Read the model definition and answer for the solid it produces. Units are mm, in the model's axes. A direction names the side the tool comes from. Give positions to 0.01 mm unless a question says otherwise; leave off trailing zeros. Order: outer loops, then holes, each group sorted by start corner. A loop starts at its lowest first (then second) coordinate and runs counter-clockwise, first axis right, second up. Notation, with made-up numbers: (38, 72.25) - (72, 72.25) arc R11 ccw to (72, 91.25) - close; hole circle Ø1 at (-8, 69). An arc over 180 degrees is marked (long way). Use a Markdown table: item, result. Add a question column.
1. Flat-ended cylindrical pins translate along their axes: P1, Ø3.5, axis at x = 14, y = 14, coming from the -Z side; P2, Ø1.3, axis at x = 13, y = 13.5, coming from the +Z side; P3, Ø1.9, axis at y = 5.5, z = -7, coming from the -X side. Find the tip coordinate at first contact, or state that the pin passes through.
2. Consider L1, parallel to Y at x = 14, z = -0.4; L2, parallel to Y at x = 14, z = -2.05; L3, parallel to X at y = -5, z = -2.25. Determine where each line is inside the solid, lowest interval first.
3. A cutting plane is placed at A-A on x = 14. Determine the outline of the cut face in (y, z), and give its area (3 significant figures).
4. Which of the six approach directions +Z, -Z, +X, -X, +Y, -Y give full straight-line access (tool end or side, diameter ignored) to faces 5 (the flat face through (-22.014, -7.678, -4.182)), 6 (the cylindrical face through (-11.43, 11.4, -1.97)), 7 (the cylindrical face through (24.22, 0.72, -9.29))?
5. A cutting plane is placed at B-B on y = -14. State how many separate pieces and enclosed holes the cut face has, and give its area (3 significant figures).
6. For a pull along Y with two mould halves and no side action, classify faces 1 (the cylindrical face through (18.4, 18.43, -1.97)), 2 (the flat face through (-21, 0, -12)), 3 (the cylindrical face through (14.176, -12.661, -3.586)), 4 (the flat face through (-14, 12.5, -1)) as released by +Y, released by -Y, zero draft, split by the parting line, or undercut.
7. A cutting plane is placed at C-C on x = -3.5. Determine the outline of the cut face in (y, z).
```python
from build123d import *

# Parameters (mm, degrees)
EXTRUDE_1_DEPTH           = 4
EXTRUDE_START             = -4
SKETCH_6_R                = 2.5000000000000004
SKETCH_6_R_2              = 2.4999999999999987
EXTRUDE_5_DEPTH           = 2.1
HOLE_WIZARD_1_D           = 2.7
HOLE_WIZARD_1_CBORE_D     = 4.5
HOLE_WIZARD_1_CBORE_DEPTH = 1
EXTRUDE_3_DEPTH           = 4
FILLET_1_R                = 2
CUT_EXTRUDE_1_DEPTH       = 2
SKETCH_14_R               = 3.150000000000003
CUT_EXTRUDE_4_DEPTH       = 0.8
EXTRUDE_6_DEPTH           = 3
SKETCH_11_R               = 2.399999999999999
EXTRUDE_7_DEPTH           = 5
FILLET_2_RADIUS           = 6
FILLET_2_LENGTH           = 3
FILLET_4_R                = 2
FILLET_6_R                = 0.5
CUT_EXTRUDE_2_DEPTH       = 0.4
CUT_EXTRUDE_3_DEPTH       = 0.4
CHAMFER_1_SIZE            = 2.5


with BuildPart() as part:
    # 草图1 → 凸台-拉伸1 (new body)
    with BuildSketch(Plane.XY):
        Polygon((19, -19), (11.999999999999977, -19), (11.000000000000004, -19), (11.000000000000002, -11.999999999999998), (11.999999999999977, -11.999999999999973), (11.999999999999977, 12.000000000000027), (-12.000000000000023, 12.000000000000023), (-12.000000000000023, -11.999999999999977), (-10.999999999999996, -12.000000000000002), (-10.999999999999996, -19), (-11.999999999999996, -19), (-19, -19), (-19, 19), (19, 19), align=None)
    extrude(amount=-EXTRUDE_1_DEPTH)

    # 草图6 → 凸台-拉伸5 (add)
    with BuildSketch(Plane.XY.offset(EXTRUDE_START)):
        with Locations((-14.000000000000115, 14.000000000000014)):
            Circle(SKETCH_6_R)
        with Locations((-14.000000000000112, -13.999999999999996)):
            Circle(SKETCH_6_R)
        with Locations((14.0000000000001, -13.99999999999998)):
            Circle(SKETCH_6_R_2)
        with Locations((14.000000000000096, 14.00000000000002)):
            Circle(SKETCH_6_R_2)
    extrude(amount=-EXTRUDE_5_DEPTH)

    # 孔1 (through all)
    with Locations(Plane.XY):
        with Locations((-14, 14), (14, -14), (14, 14), (-14, -14), (0, 0), (0.008296822, -0.048065229)):
            CounterBoreHole(HOLE_WIZARD_1_D / 2, HOLE_WIZARD_1_CBORE_D / 2, HOLE_WIZARD_1_CBORE_DEPTH)

    # 草图5 → 凸台-拉伸3 (add)
    with BuildSketch(Plane.ZY.offset(19)):
        Polygon((-12.000000000000004, -19.000000000000007), (-4.47e-15, -19.000000000000004), (-3.7e-16, 18.999999999999996), (-12.000000000000004, 18.999999999999993), align=None)
    extrude(amount=EXTRUDE_3_DEPTH)

    # 圆角1
    # the kernel refuses this fillet: 2 mm, written as the material it adds along each edge
    with BuildSketch(Plane(origin=(11.999999999999977, 12.000000000000027, 0), x_dir=(-1, 0, 0), z_dir=(0, 0, -1)), Plane(origin=(-12.000000000000023, 12.000000000000023, 0), x_dir=(0, -1, 0), z_dir=(0, 0, -1))) as fillet_1_piece_1:
        with BuildLine():
            CenterArc((FILLET_1_R, -FILLET_1_R), FILLET_1_R, 90, 90)
            Line((0, -FILLET_1_R), (0, 0))
            Line((0, 0), (FILLET_1_R, 0))
        make_face()
    extrude(amount=4)
    with BuildSketch(Plane(origin=(11.999999999999977, -11.999999999999973, 0), x_dir=(0, 1, 0), z_dir=(0, 0, -1))) as fillet_1_piece_2:
        with BuildLine():
            CenterArc((1.7320508075689318, -2), FILLET_1_R, 90, 60.00000000000051)
            Line((4.619e-14, -1.000000000000016), (0, 0))
            Line((0, 0), (1.7320508075689318, 0))
        make_face()
    extrude(amount=4)
    with BuildSketch(Plane(origin=(-12.000000000000023, -11.999999999999977, 0), x_dir=(1, 4.796e-14, 0), z_dir=(0, 0, -1))) as fillet_1_piece_3:
        with BuildLine():
            CenterArc((2.000000000000083, -1.7320508075688679), FILLET_1_R, 120.00000000000053, 60.00000000000222)
            Line((8.307e-14, -1.7320508075689638), (0, 0))
            Line((0, 0), (1.0000000000000675, 0))
        make_face()
    extrude(amount=4)
    # the kernel refuses this fillet: 2 mm, written as the material it takes off along each edge
    with BuildSketch(Plane(origin=(19, -19, 5), x_dir=(-1, 0, 0), z_dir=(0, 0, -1)), Plane(origin=(19, 19, 5), x_dir=(0, -1, 0), z_dir=(0, 0, -1))) as fillet_1_2_piece_1:
        with BuildLine():
            CenterArc((FILLET_1_R, FILLET_1_R), FILLET_1_R, 180, 90)
            Line((0, FILLET_1_R), (0, 0))
            Line((0, 0), (FILLET_1_R, 0))
        make_face()
    extrude(amount=14, mode=Mode.SUBTRACT)
    with BuildSketch(Plane(origin=(-23, -19.000000000000007, -17.000000000000004), x_dir=(1, 3.55e-15, 0), z_dir=(0, 3e-16, 1))) as fillet_1_2_piece_2:
        with BuildLine():
            CenterArc((FILLET_1_R, FILLET_1_R), FILLET_1_R, 180, 89.99999999999977)
            Line((7.11e-15, FILLET_1_R), (0, 0))
            Line((0, 0), (FILLET_1_R, 0))
        make_face()
    extrude(amount=22, mode=Mode.SUBTRACT)
    with BuildSketch(Plane(origin=(-23, 18.999999999999996, 5), x_dir=(1, 3.55e-15, 0), z_dir=(0, -3e-16, -1))) as fillet_1_2_piece_3:
        with BuildLine():
            CenterArc((FILLET_1_R, FILLET_1_R), FILLET_1_R, 180, 90.00000000000023)
            Line((-7.11e-15, FILLET_1_R), (0, 0))
            Line((0, 0), (FILLET_1_R, 0))
        make_face()
    extrude(amount=22.000000000000004, mode=Mode.SUBTRACT)

    # 草图9 → 切除-拉伸1 (cut)
    with BuildSketch(Plane(origin=(-23, 0, -24), x_dir=(0, 0, -1), z_dir=(1, 0, 0))):
        with BuildLine():
            Line((-19.497620553954647, -15.010679125349048), (-20.147001897982854, -0.1374010702007968))
            ThreePointArc((-20.147001897982854, -0.1374010702007968), (-16.999999999999996, 3.149999999999999), (-13.852998102017144, -0.13740107020079845))
            Line((-13.852998102017144, -0.13740107020079845), (-14.50237944604535, -15.01067912534905))
            ThreePointArc((-14.50237944604535, -15.01067912534905), (-16.999999999999993, -17.401630656935822), (-19.497620553954647, -15.010679125349048))
        make_face()
    cut_extrude_1 = extrude(amount=CUT_EXTRUDE_1_DEPTH, mode=Mode.SUBTRACT)

    # 镜向2: 切除-拉伸1 across plane
    add(cut_extrude_1.mirror(Plane.ZX), mode=Mode.SUBTRACT)

    # 草图14 → 切除-拉伸4 (cut)
    with BuildSketch(Plane.ZY.offset(20.999999999999996)):
        with Locations((-7.000000000000003, -6.1e-16)):
            Circle(SKETCH_14_R)
    extrude(amount=-CUT_EXTRUDE_4_DEPTH, mode=Mode.SUBTRACT)

    # 草图10 → 凸台-拉伸6 (add)
    with BuildSketch(Plane(origin=(19, 0, 0), x_dir=(0, 0, -1), z_dir=(1, 0, 0))):
        Polygon((1.59e-15, 6), (12.000000000000002, 6.000000000000002), (12.000000000000002, -6.000000000000002), (1.59e-15, -6), align=None)
    extrude(amount=EXTRUDE_6_DEPTH)

    # 草图11 → 凸台-拉伸7 (add)
    with BuildSketch(Plane(origin=(22, 0, 0), x_dir=(0, 0, -1), z_dir=(1, 0, 0))):
        with Locations((7.000000000000001, 0)):
            Circle(SKETCH_11_R)
    extrude(amount=EXTRUDE_7_DEPTH)

    # 圆角2: full round fillet: the end face becomes a half cylinder, R = half its width
    fillet_2_face = Plane((20.5, 0, -12), x_dir=(-1, 0, 0), z_dir=(0, 0, -1))  # on the end face: x along it, z out of the body
    fillet_2_slab = fillet_2_face.offset(-FILLET_2_RADIUS / 2) * Box(FILLET_2_LENGTH, 2 * FILLET_2_RADIUS, FILLET_2_RADIUS, mode=Mode.PRIVATE)  # the body's end, R deep
    fillet_2_round = Plane((20.5, 0, -6), x_dir=(0, 0, -1), z_dir=(-1, 0, 0)) * Cylinder(FILLET_2_RADIUS, FILLET_2_LENGTH, mode=Mode.PRIVATE)  # its axis R under the face
    add(fillet_2_slab - fillet_2_round, mode=Mode.SUBTRACT)

    # 圆角4
    fillet_4_edges = [part.edges().sort_by_distance(p)[0] for p in [
        (19, -6, -2.0000000000000018),
        (19, 6, -2.000000000000001),
    ]]
    fillet(fillet_4_edges, radius=FILLET_4_R)

    # 圆角6
    fillet_6_edges = [part.edges().sort_by_distance(p)[0] for p in [
        (27, 2.9e-16, -4.600000000000001),
    ]]
    fillet(fillet_6_edges, radius=FILLET_6_R)

    # 草图12 → 切除-拉伸2 (cut)
    with BuildSketch(Plane.ZY.offset(-19)):
        with BuildLine():
            Line((-4, 6.000000000000001), (-5.999999999999998, 6.000000000000001))
            ThreePointArc((-5.999999999999998, 6.000000000000001), (-12, 7.3e-16), (-6, -6.000000000000001))
            Line((-6, -6.000000000000001), (-4, -6.000000000000001))
            Line((-4, -6.000000000000001), (-4, 6.000000000000001))
        make_face()
    extrude(amount=-CUT_EXTRUDE_2_DEPTH, mode=Mode.SUBTRACT)

    # 草图13 → 切除-拉伸3 (cut)
    with BuildSketch(Plane(origin=(-19, 0, 0), x_dir=(0, 0, -1), z_dir=(1, 0, 0))):
        Polygon((12.000000000000004, -19.000000000000007), (12.000000000000004, 18.999999999999993), (4, 19), (4, -19.000000000000004), align=None)
    extrude(amount=-CUT_EXTRUDE_3_DEPTH, mode=Mode.SUBTRACT)

    # 倒角1
    chamfer_1_edges = [part.edges().sort_by_distance(p)[0] for p in [
        (-19.4, 0, -4),
        (19.4, 0, -4),
    ]]
    chamfer(chamfer_1_edges, length=CHAMFER_1_SIZE)


solid = part.part
```
Output values:
| question | item | result |
|---|---|---|
| 1 | P1 | z = -6.1 |
| 1 | P2 | z = -1 |
| 1 | P3 | x = -21 |
| 2 | L1 | -19 to -16.25, -11.75 to 11.75, 16.25 to 19 |
| 2 | L2 | -19 to -15.35, -12.65 to 12.65, 15.35 to 19 |
| 2 | L3 | -23 to -12, 12 to 22 |
| 3 | outline | (-19, -4) - (-16.5, -4) - (-16.5, -6.1) - (-15.35, -6.1) - (-15.35, -1) - (-16.25, -1) - (-16.25, 0) - (-19, 0) - close; (-12.65, -6.1) - (-11.5, -6.1) - (-11.5, -4) - (11.5, -4) - (11.5, -6.1) - (12.65, -6.1) - (12.65, -1) - (11.75, -1) - (11.75, 0) - (-11.75, 0) - (-11.75, -1) - (-12.65, -1) - close; (15.35, -6.1) - (16.5, -6.1) - (16.5, -4) - (19, -4) - (19, 0) - (16.25, 0) - (16.25, -1) - (15.35, -1) - close |
| 3 | area | 136 mm² |
| 4 | face 5 | -X |
| 4 | face 6 | +Z, -Z |
| 4 | face 7 | +X |
| 5 | separate pieces | 4 |
| 5 | enclosed holes | 0 |
| 5 | area | 86.2 mm² |
| 6 | face 1 | released by +Y |
| 6 | face 2 | zero draft |
| 6 | face 3 | undercut |
| 6 | face 4 | undercut |
| 7 | outline | (12, -4) - (19, -4) - (19, 0) - (12, 0) - close |
